```python
from build123d import *

# Parameters (mm, degrees)
SKETCH1_W           = 58.5
SKETCH1_H           = 49
SKETCH1_R           = 3.1
BOSS_EXTRUDE1_DEPTH = 1.5
BOSS_EXTRUDE2_DEPTH = 49
CUT_EXTRUDE1_DEPTH  = 2
CHAMFER2_SIZE       = 0.2
CUT_EXTRUDE3_DEPTH  = 64.549193543
CHAMFER3_SIZE       = 2


with BuildPart() as part:
    # Sketch1 → Boss-Extrude1 (new body)
    with BuildSketch(Plane(origin=(0, 0, 0), x_dir=(1, 0, 0), z_dir=(0, 1, 0))):
        Rectangle(SKETCH1_W, SKETCH1_H)
        with Locations(Location((0, 0, 0), (0, 0, 270))):
            Circle(SKETCH1_R, mode=Mode.SUBTRACT)
    extrude(amount=BOSS_EXTRUDE1_DEPTH)

    # Sketch2 → Boss-Extrude2 (add)
    with BuildSketch(Plane(origin=(0, 0, -24.5), x_dir=(-1, 0, 0), z_dir=(0, 0, -1))):
        Polygon((-29.25, 1.5), (29.25, 1.5), (29.25, 2.5), (28.08, 4), (26.91, 2.5), (25.74, 4), (24.57, 2.5), (23.4, 4), (22.23, 2.5), (21.06, 4), (19.89, 2.5), (18.72, 4), (17.55, 2.5), (16.38, 4), (15.21, 2.5), (14.04, 4), (12.87, 2.5), (11.7, 4), (10.53, 2.5), (9.36, 4), (8.19, 2.5), (7.02, 4), (5.85, 2.5), (4.68, 4), (3.51, 2.5), (2.34, 4), (1.17, 2.5), (0, 4), (-1.17, 2.5), (-2.34, 4), (-3.51, 2.5), (-4.68, 4), (-5.85, 2.5), (-7.02, 4), (-8.19, 2.5), (-9.36, 4), (-10.53, 2.5), (-11.7, 4), (-12.87, 2.5), (-14.04, 4), (-15.21, 2.5), (-16.38, 4), (-17.55, 2.5), (-18.72, 4), (-19.89, 2.5), (-21.06, 4), (-22.23, 2.5), (-23.4, 4), (-24.57, 2.5), (-25.74, 4), (-26.91, 2.5), (-28.08, 4), (-29.25, 2.5), align=None)
    extrude(amount=-BOSS_EXTRUDE2_DEPTH)

    # Sketch3 → Cut-Extrude1 (cut)
    with BuildSketch(Plane(origin=(0, 0, 0), x_dir=(-1, 0, 0), z_dir=(0, -1, 0))):
        with BuildLine():
            Line((-1.75, -2.558808316), (-1.75, -5))
            Line((-1.75, -5), (1.75, -5))
            Line((1.75, -5), (1.75, -2.558808316))
            ThreePointArc((1.75, -2.558808316), (0, 3.1), (-1.75, -2.558808316))
        make_face()
    extrude(amount=-CUT_EXTRUDE1_DEPTH, mode=Mode.SUBTRACT)

    # Chamfer2
    chamfer2_edges = [part.edges().sort_by_distance(p)[0] for p in [
        (0, 0, -3.1),
    ]]
    chamfer(chamfer2_edges, length=CHAMFER2_SIZE)

    # Sketch4 → Cut-Extrude3 (cut, through all)
    with BuildSketch(Plane(origin=(29.25, 0, 0), x_dir=(0, 0, -1), z_dir=(1, 0, 0))):
        with BuildLine():
            Line((-23.75, 4), (-24.5, 4))
            Line((-24.5, 4), (-24.5, 3.25))
            ThreePointArc((-24.5, 3.25), (-24.280330086, 3.780330086), (-23.75, 4))
        make_face()
    cut_extrude3 = extrude(amount=-CUT_EXTRUDE3_DEPTH, mode=Mode.SUBTRACT)

    # Mirror1: Cut-Extrude3 across plane
    add(cut_extrude3.mirror(Plane.XY), mode=Mode.SUBTRACT)

    # Chamfer3
    chamfer3_edges = [part.edges().sort_by_distance(p)[0] for p in [
        (0, 0, 5),
    ]]
    chamfer(chamfer3_edges, length=CHAMFER3_SIZE - 0.0001)  # a hair under: the kernel refuses the full size


solid = part.part
```
Verification items for the finished model (mm, model axes). A direction names the side the tool comes from. Coordinates: 2 decimals unless noted, no trailing zeros. Put each result on its own line as item: value.
1. Thickness scan on line 1 (X direction, y = 0.8, z = 0); line 2 (Y direction, x = 13.5, z = -8.5); line 3 (Z direction, x = 0, y = 1). Record the ranges inside material, lowest first.
Result set:
line 1: x = -29.25 to -3.1, 3.1 to 29.25
line 2: y = 0 to 3.31
line 3: z = -24.5 to -3.1, 6 to 24.5
2. Gauge pin test, flat ends, axial feed: P1, Ø3, axis at x = 1, z = 2.5, coming from the -Y side; P2, Ø8, axis at x = 0, z = 0, coming from the +Y side. Record the tip position at first contact, or that the pin passes through.
Result set:
P1: stops at y = 0
P2: stops at y = 4
3. Mould release check, pull along X, two halves, no side actions. Record for faces 4 (the face through (20.467, 3.24, -0.343)), 5 (the face through (28.657, 3.261, -0.343)), 6 (the face through (0, 2, 24.5)): pulls with the +X half, pulls with the -X half, needs draft (parallel to the pull), parting line crosses it, or undercut.
Result set:
face 4: undercut
face 5: pulls with the +X half
face 6: needs draft
4. Tool access check on faces 1 (the face through (5.257, 3.26, -0.343)), 2 (the face through (0, 2, 1)), 3 (the face through (0, 2, -24.5)). Record the directions out of +Z, -Z, +X, -X, +Y, -Y that give a thin tool (end or side, any length) a straight path to the whole face; none if there is none.
Result set:
face 1: +Z, -Z, +Y
face 2: -Y
face 3: -Z, +X, -X, +Y, -Y
